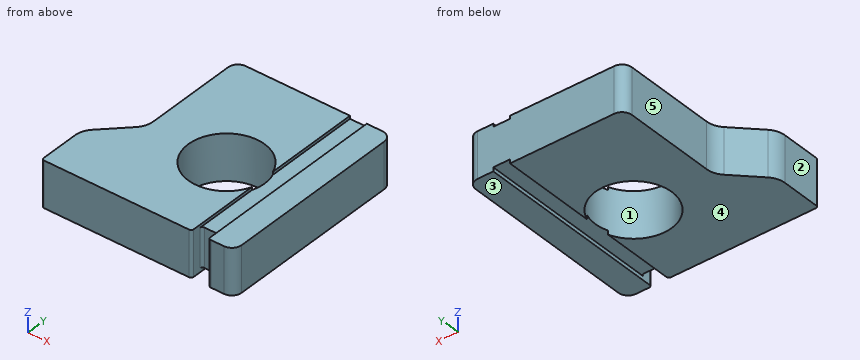
Autodesk Fusion 360 part; units mm, degrees
sketch "Skizze1" plane through (0, 0, 0) normal (0, 0, 1) x (1, 0, 0)
  line L0 (0, 19.86) -> (15.85, 19.86)
  line L1 (15.85, 19.86) -> (15.85, 0)
  circle A0 centre (7.925, 8.925) radius 3.925 construction
  line L2 (-3.65, 5) -> (15.85, 5) construction
  line L3 (4, 19.86) -> (4, 0) construction
  line L4 (0, 0) -> (4, 0)
  line L5 (4, 0) -> (11.57, 0)
  line L6 (11.85, 1.3) -> (13.27, 1.3)
  line L7 (13.27, 1.3) -> (13.27, 0)
  line L8 (13.27, 0) -> (15.85, 0)
  line L9 (11.85, 19.86) -> (11.85, 1.3) construction
  line L10 (11.57, 0) -> (11.57, 1.3)
  line L11 (11.57, 1.3) -> (11.85, 1.3)
  line L12 (11.57, 0) -> (13.27, 0) construction
  line L13 (0, 0) -> (-3.65, 0)
  line L14 (-3.65, 0) -> (-3.65, 5)
  line L15 (-3.65, 5) -> (0, 8.65)
  line L16 (0, 8.65) -> (0, 19.86)
  line L17 (0, 0) -> (0, 8.65) construction
  circle A1 centre (7.925, 8.875) radius 3.875
  line L18 (7.925, 8.875) -> (7.925, 8.925) construction
  dimension "d1" = 7.85
  dimension "d2" = 5
  dimension "d3" = 19.86
  dimension "d4" = 4
  dimension "d5" = 0.28
  dimension "d6" = 1.42
  dimension "d7" = 1.3
  dimension "d8" = 4
  dimension "d9" = 7.65
  dimension "d10" = 5
  dimension "d11" = 135
  dimension "d27" = 7.75
extrude "Extrusion1" add sketch "Skizze1" along normal blind 4.65
sketch "Skizze2" plane through (0, 0, 4.65) normal (0, 0, 1) x (-1, 0, 0)
  line L0 (3.65, 0) -> (-11.57, 0)
  line L1 (-11.57, 0) -> (-11.57, -1.3)
  line L2 (-11.57, -1.3) -> (-13.27, -1.3)
  line L3 (-13.27, -1.3) -> (-13.27, 0)
  line L4 (-13.27, 0) -> (-15.85, 0)
  line L5 (-15.85, 0) -> (-15.85, -19.86)
  line L6 (-15.85, -19.86) -> (0, -19.86)
  line L7 (0, -19.86) -> (0, -8.65)
  line L8 (0, -8.65) -> (3.65, -5)
  line L9 (3.65, -5) -> (3.65, 0)
  line L10 (-11.57, -1.3) -> (-11.57, -19.86)
  line L11 (-11.57, -1.3) -> (-13.27, -1.3)
  line L12 (-13.27, -1.3) -> (-13.27, -19.86)
  line L13 (-13.27, -19.86) -> (-11.57, -19.86)
  circle A0 centre (-7.925, -8.875) radius 3.875
extrude "Extrusion2" cut sketch "Skizze2" against normal blind 0.3 contours L2 L6 L10 L11 L12 L13 A0
extrude "Extrusion3" cut sketch "Skizze2" along normal blind 0.4 from surface at -4.65 contours L2 L6 L10 L11 L12 L13 A0
fillet "Abrundung1" radius 1 3 edges at (0, 19.86, 2.325) (15.85, 19.86, 2.325) (15.85, 0, 2.325)
fillet "Abrundung2" radius 0.25 1 edges at (-3.65, 0, 2.325)
fillet "Abrundung3" radius 2 2 edges at (-3.65, 5, 2.325) (0, 8.65, 2.325)
fillet "Abrundung4" radius 0.25 4 edges at (13.27, 0, 2.325) (11.57, 0, 2.325) (11.57, 1.3, 2.375) (13.27, 1.3, 2.375)
equation "d1 = 7.6 mm + 0.25 mm"
equation "d3 = 14 mm + 5.3 mm + 1.2 mm - 0.5 mm - 0.1 mm - 0.04 mm"
Model file for the job. Use its own axes, mm. Face numbers are marked on the shaded views. A direction names the side the tool comes from. Give positions to 0.01 mm unless a question says otherwise; leave off trailing zeros. Loops run counter-clockwise (first coordinate to the right, second up) from the corner with the lowest first, then second, coordinate; pieces in that order, holes last. Notation, with made-up numbers: (-23, 32) -> (6, 32) arc R26 ccw to (6, 53) -> close; hole circle Ø4 at (20, 6). An arc over 180 degrees is marked (long way). Use a Markdown table: item, result. Add a question column.
(1) Slice it at D-D on z = 1.4. List the corners of the cut face in (x, y) (3 decimals).
(2) Drop flat-ended pins along their axis: pin 1 Ø1.9 at (x, y) = (12, 14.5) entering from -Z; pin 2 Ø1.5 at (y, z) = (6, 2.5) entering from -X; pin 3 Ø1.3 at (x, z) = (12.5, 3) entering from -Y; pin 4 Ø0.5 at (x, y) = (12.5, 9) entering from +Z. Give the stop position or say it passes through.
(3) Mould opens along X. For the marked faces 1, 2 and 3 say: +X half, -X half, draft (parallel to the pull), parting line (faces both ways), or undercut.
(4) Wall check: line 1 along X through (y, z) = (14.25, 1.55); line 2 along Y through (x, z) = (4.75, 2.2); line 3 along X through (y, z) = (5.75, 3.05). Give the ranges that are in metal, low to high.
(5) Slice it at A-A on y = 18. List the corners of the cut face in (x, z).
(6) Slice it at B-B on x = 9.75. List the corners of the cut face in (y, z).
(7) Slice it at C-C on y = 12.5. List the corners of the cut face in (x, z), and give its area (3 significant figures).
(8) Tool access for the marked faces 4 and 5: list every direction of +Z, -Z, +X, -X, +Y, -Y with a clear straight run to the whole face (end or side of a thin tool).
Filled sheet:
| question | item | result |
|---|---|---|
| 1 | outline | (-3.65, 0.25) arc R0.25 ccw to (-3.4, 0) -> (11.32, 0) arc R0.25 ccw to (11.57, 0.25) -> (11.57, 1.05) arc R0.25 cw to (11.82, 1.3) -> (13.02, 1.3) arc R0.25 cw to (13.27, 1.05) -> (13.27, 0.25) arc R0.25 ccw to (13.52, 0) -> (14.85, 0) arc R1 ccw to (15.85, 1) -> (15.85, 18.86) arc R1 ccw to (14.85, 19.86) -> (1, 19.86) arc R1 ccw to (0, 18.86) -> (0, 9.478) arc R2 cw to (-0.586, 8.064) -> (-3.064, 5.586) arc R2 ccw to (-3.65, 4.172) -> close; hole circle Ø7.75 at (7.925, 8.875) |
| 2 | pin 1 | z = 0 |
| 2 | pin 2 | x = -3.33 |
| 2 | pin 3 | y = 1.26 |
| 2 | pin 4 | z = 4.35 |
| 3 | face 1 | undercut |
| 3 | face 2 | -X half |
| 3 | face 3 | draft |
| 4 | line 1 | 0 to 15.85 |
| 4 | line 2 | 0 to 6.65, 11.1 to 19.86 |
| 4 | line 3 | -2.9 to 5.63, 10.22 to 15.85 |
| 5 | outline | (0, 0) -> (11.57, 0) -> (11.57, 0.4) -> (13.27, 0.4) -> (13.27, 0) -> (15.85, 0) -> (15.85, 4.65) -> (13.27, 4.65) -> (13.27, 4.35) -> (11.57, 4.35) -> (11.57, 4.65) -> (0, 4.65) -> close |
| 6 | outline | (0, 0) -> (5.46, 0) -> (5.46, 4.65) -> (0, 4.65) -> close; (12.29, 0) -> (19.86, 0) -> (19.86, 4.65) -> (12.29, 4.65) -> close |
| 7 | outline | (0, 0) -> (6.56, 0) -> (6.56, 4.65) -> (0, 4.65) -> close; (9.29, 0) -> (11.57, 0) -> (11.57, 0.4) -> (13.27, 0.4) -> (13.27, 0) -> (15.85, 0) -> (15.85, 4.65) -> (13.27, 4.65) -> (13.27, 4.35) -> (11.57, 4.35) -> (11.57, 4.65) -> (9.29, 4.65) -> close |
| 7 | area | 59.8 mm2 |
| 8 | face 4 | -Z, +X, -X, +Y, -Y |
| 8 | face 5 | +Z, -Z, -X, +Y |
